Autodesk Inventor part; units mm, degrees
ref_plane "YZ Plane" through (0, 0, 0) normal (1, 0, 0) x (0, 1, 0)
ref_plane "XZ Plane" through (0, 0, 0) normal (0, 1, 0) x (-1, 0, 0)
ref_plane "XY Plane" through (0, 0, 0) normal (0, 0, 1) x (1, 0, 0)
sketch "Sketch1" plane through (0, 0, 0) normal (0, 0, 1) x (1, 0, 0)
  line L0 (0, 0) -> (176.8, 0)
  line L1 (176.8, 0) -> (176.8, 304.8)
  line L2 (176.8, 304.8) -> (0, 304.8)
  line L3 (0, 304.8) -> (0, 0)
  dimension "d1" = 176.8
  dimension "d2" = 304.8
extrude "Extrusion1" add sketch "Sketch1" along normal blind 12.7
sketch "Sketch2" plane through (0, 0, 12.7) normal (0, 0, 1) x (1, 0, 0)
  line L0 (0, 0) -> (176.8, 0)
  line L1 (0, 304.8) -> (0, 0)
  point P0 (8, 11)
  point P1 (8, 51)
  point P2 (8, 91)
  point P3 (8, 131)
  dimension "d5" = 40
  dimension "d6" = 40
  dimension "d7" = 40
  dimension "d8" = 11
  dimension "d9" = 8
hole "Hole1" at (8, 11, 12.7) at (8, 51, 12.7) at (8, 91, 12.7) at (8, 131, 12.7) direction (0, 0, -1) diameter 6.604 end through all
pattern_linear "Rectangular Pattern1" count 2 spacing 162.8 along (0, 1, 0) count 2 spacing 161 along (1, 0, 0) of "Hole1"
properties part number "actuatorMount" material "Aluminum 6061"
The model under review builds one solid part; all positions refer to its coordinate system, in mm. Round coordinates to 2 decimals unless told otherwise and drop trailing zeros. Write each loop counter-clockwise with the first axis right and the second up, starting at its lowest first coordinate (ties: lowest second). Pieces come first, ordered by that corner, then holes. Notation, with made-up numbers: M 10.25,9 L 22.25,9 A21 cw 22.25,23 Z; hole C 64,30.25 d4. An arc over 180 degrees is marked long. Use CSV: the item, a comma, the result in double quotes. Start each with the question number.
(1) For line 1 along X through (y, z) = (173.8, 5.5), list the stretches that pass through material, from the lowest coordinate up.
(2) Clearance check with a flat-ended pin moving along its axis: P1, Ø5.5, axis at x = 169, y = 51, coming from the -Z side. State where the tip first meets the part, or that it passes through.
(3) We need section B-B, the plane x = 8. State how many separate pieces and enclosed holes the cut face has, then the cut area to 3 significant figures.
(4) The part is to be moulded in two halves that separate along Y. For faces 1 (the face through (176.8, 150, 6)), 2 (the face through (168.9, 297.1, 6.3)), 3 (the face through (87, 0, 6)), say which applies: +Y half, -Y half, draft (parallel to the pull), parting line (faces both ways), or undercut.
(5) We need section A-A, the plane y = 131. State the section outline as (x, z) points.
Findings:
1,line 1,"0 to 4.7, 11.3 to 165.7, 172.3 to 176.8"
2,P1,"through"
3,separate pieces,"9"
3,enclosed holes,"0"
3,area,"3,200 mm^2"
4,face 1,"draft"
4,face 2,"undercut"
4,face 3,"-Y half"
5,outline,"M 0,0 L 4.7,0 L 4.7,12.7 L 0,12.7 Z; M 11.3,0 L 165.7,0 L 165.7,12.7 L 11.3,12.7 Z; M 172.3,0 L 176.8,0 L 176.8,12.7 L 172.3,12.7 Z"
